```python
from build123d import *

# Parameters (mm, degrees)
F0_R     = 6.35
F1_DEPTH = 0.127
F3_R     = 5.084665
F3_R_2   = 3.808429
F4_DEPTH = 1.27
F3_R_3   = 2.542971
F5_DEPTH = 2.54
F3_R_4   = 1.272508
F6_DEPTH = 3.81
F7_DEPTH = 5.08
F8_R     = 3.175
F9_DEPTH = 73.66


with BuildPart() as f1:
    # F0 (on Front) → F1 (new body)
    with BuildSketch(Plane.XZ):
        Circle(F0_R)
    extrude(amount=F1_DEPTH)

    # F3 (on face) → F4 (join)
    with BuildSketch(Plane.XZ.offset(0.127)):
        Circle(F3_R)
        Circle(F3_R_2, mode=Mode.SUBTRACT)
    extrude(amount=F4_DEPTH)

    # F3 (on face) → F5 (join)
    with BuildSketch(Plane.XZ.offset(0.127)):
        Circle(F3_R_2)
        Circle(F3_R_3, mode=Mode.SUBTRACT)
    extrude(amount=F5_DEPTH)

    # F3 (on face) → F6 (join)
    with BuildSketch(Plane.XZ.offset(0.127)):
        Circle(F3_R_3)
        Circle(F3_R_4, mode=Mode.SUBTRACT)
    extrude(amount=F6_DEPTH)

    # F3 (on face) → F7 (join)
    with BuildSketch(Plane.XZ.offset(0.127)):
        Circle(F3_R_4)
    extrude(amount=F7_DEPTH)

    # F8 (on face) → F9 (join)
    with BuildSketch(Plane.XZ):
        Circle(F8_R)
    extrude(amount=-F9_DEPTH)


solid = f1.part
```
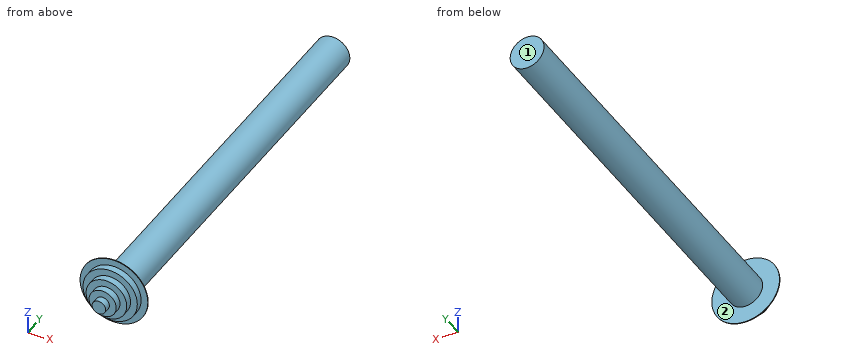
Source: CAD feature listing. Evaluate the final solid. Frame: model axes, mm. Face numbers are marked on the shaded views. A direction names the side the tool comes from. Round coordinates to 2 decimals unless told otherwise and drop trailing zeros. Loops run counter-clockwise (first coordinate to the right, second up) from the corner with the lowest first, then second, coordinate; pieces in that order, holes last. Notation, with made-up numbers: M 43,30 L 81,30 A15 cw 81,37 Z; hole C 74,79 d5. An arc over 180 degrees is marked long. Use a Markdown table: item, result. Add a question column.
1. Set-up query: the marked faces 1 and 2. Return all of +Z, -Z, +X, -X, +Y, -Y with unobstructed straight access to the full face (end or side cutting, diameter ignored); none if empty.
2. Cut plane C-C, the plane y = 55.5. Output: boundary loops of the cut face in (x, z) (3 decimals).
3. Contact query for flat-ended pins moving along their axis: pin 1 (6 mm diameter, centred on y = 4.5, z = -2.5, fed in from +X) (3 decimals); pin 2 (6 mm diameter, centred on x = 2, y = 12, fed in from -Z) (3 decimals); pin 3 (1.5 mm diameter, centred on x = -4, z = -2, fed in from +Y). Output: stop coordinate, or through.
4. Ray query, line 1 along X through (y, z) = (15.5, 0.25); line 2 along Y through (x, z) = (-1.5, -4); line 3 along Y through (x, z) = (2.75, 0.25). Return the intervals inside material, ascending. Write a range as [from, to].
Solution:
| question | item | result |
|---|---|---|
| 1 | face 1 | +Z, -Z, +X, -X, +Y |
| 1 | face 2 | +Y |
| 2 | outline | C 0,0 d6.35 |
| 3 | pin 1 | stops at x = 3.175 |
| 3 | pin 2 | stops at z = -3.175 |
| 3 | pin 3 | stops at y = 0 |
| 4 | line 1 | x = [-3.17, 3.17] |
| 4 | line 2 | y = [-1.4, 0] |
| 4 | line 3 | y = [-2.67, 73.66] |
